from build123d import *

# Parameters (mm, degrees)
SKETCH1_W = 12.7
SKETCH1_H = 101.6


with BuildPart() as part:
    # Sketch1 → Revolve1 (revolve)
    with BuildSketch(Plane(origin=(0, 0, 0), x_dir=(1, 0, 0), z_dir=(0, 1, 0))):
        with Locations((6.35, 50.8)):
            Rectangle(SKETCH1_W, SKETCH1_H)
    revolve(axis=Axis((0, 0, 0), (0, 0, -1)))

    # Sketch5 → Cut-Revolve1 (revolve, cut)
    with BuildSketch(Plane(origin=(0, 25.4, 0), x_dir=(-1, 0, 0), z_dir=(0, -1, 0))):
        with BuildLine():
            Line((22.718491956, 6.35), (-23.001508044, 6.35))
            ThreePointArc((-23.001508044, 6.35), (-0.141508044, -16.51), (22.718491956, 6.35))
        make_face()
    revolve(axis=Axis((-22.718491956, 25.4, -6.35), (1, 0, 0)), mode=Mode.SUBTRACT)

    # Sketch6 → Cut-Revolve2 (revolve, cut)
    with BuildSketch(Plane(origin=(0, -25.4, 0), x_dir=(1, 0, 0), z_dir=(0, 1, 0))):
        with BuildLine():
            Line((22.718491956, 6.35), (-23.001508044, 6.35))
            ThreePointArc((-23.001508044, 6.35), (-0.141508044, -16.51), (22.718491956, 6.35))
        make_face()
    revolve(axis=Axis((22.718491956, -25.4, -6.35), (-1, 0, 0)), mode=Mode.SUBTRACT)


solid = part.part
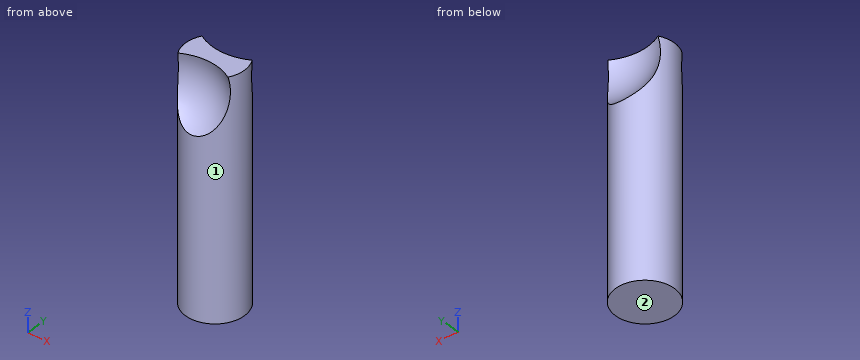
Work out the finished part from the listing and answer in its coordinate system (mm). Face numbers are marked on the shaded views. Give positions to 0.01 mm unless a question says otherwise; leave off trailing zeros. Order: outer loops, then holes, each group sorted by start corner. A loop starts at its lowest first (then second) coordinate and runs counter-clockwise, first axis right, second up. Notation, with made-up numbers: (39.5, 85) - (95.5, 85) arc R27 ccw to (95.5, 102) - close; hole circle Ø3 at (-4, 79.5). An arc over 180 degrees is marked (long way). Answer as CSV lines item,"result". Start each with the question number.
Q1. The part is cut by section B-B (z = -84). Write down the section's boundary in (x, y), then the cut area to 3 significant figures.
Q2. Given pin 1 Ø4 at (y, z) = (-3.5, -42) entering from -X; pin 2 Ø5 at (y, z) = (8, -56.5) entering from -X; pin 3 Ø4 at (x, z) = (-3, -12) entering from -Y, each flat-ended and moving along its own axis, determine where each tip first touches the part or whether it passes through.
Q3. Find the intervals of material crossed by L1, parallel to X at y = 0.5, z = -76.5; L2, parallel to Y at x = 9, z = -76; L3, parallel to Y at x = 0.75, z = -31, in increasing order. Write a range as [from, to].
Q4. The part is cut by section C-C (y = -4). Write down the section's boundary in (x, z).
Q5. The mould has two halves that part along X. Classify the marked faces 1 and 2: +X half, -X half, draft (parallel to the pull), parting line (faces both ways), or undercut.
Q6. The part is cut by section A-A (x = -8). Write down the section's boundary in (y, z).
Check result:
1,outline,"circle Ø25.4 at (0, 0)"
1,area,"507 mm²"
2,pin 1,"stops at x = -12.61"
2,pin 2,"stops at x = -11.45"
2,pin 3,"stops at y = -4.11"
3,L1,"x = [-12.69, 12.69]"
3,L2,"y = [-8.96, 8.96]"
3,L3,"y = [-12.68, 12.68]"
4,outline,"(-12.05, -101.6) - (12.05, -101.6) - (12.05, 0) - (4.79, 0) arc R8.04 cw (long way) to (-5.07, 0) - (-12.05, 0) - close"
5,face 1,"parting line"
5,face 2,"draft"
6,outline,"(-9.86, -101.6) - (9.86, -101.6) - (9.86, -21.01) arc R21.36 cw to (5, 0) - (-4.89, 0) arc R21.47 cw to (-9.86, -21.16) - close"
